Input: part model. Units: mm. Frame: model coordinates. A direction names the side the tool comes from. Coordinates: 2 decimals unless noted, no trailing zeros. Write each loop counter-clockwise with the first axis right and the second up, starting at its lowest first coordinate (ties: lowest second). Pieces come first, ordered by that corner, then holes. Notation, with made-up numbers: M 54,54.25 L 90,54.25 A25 ccw 90,81.25 Z; hole C 12.5,-5.75 d10. An arc over 180 degrees is marked long. Write each question's results on one line, items separated by ' | '. Start each with the question number.
1. First-contact query: pin 1 (4 mm diameter, centred on x = 10, y = -19, fed in from +Z); pin 2 (2.5 mm diameter, centred on x = 5.74, z = -24.03, fed in from -Y); pin 3 (8 mm diameter, centred on x = 16.5, y = -17.5, fed in from -Z); pin 4 (8 mm diameter, centred on y = -20.5, z = -42.5, fed in from +X). Flat tips, straight axial feed; report the tip coordinate or a pass-through.
2. Set-up query: faces 4 (the flat face through (-19.264, -17, -36)), 5 (the flat face through (0, -12, -35.632)), 6 (the flat face through (0, -14, -33.632)). Return all of +Z, -Z, +X, -X, +Y, -Y with unobstructed straight access to the full face (end or side cutting, diameter ignored); none if empty.
3. Pull-direction query (Z, two-part tool) for faces 1 (the flat face through (1, -26, -46)), 2 (the cylindrical face through (6.412, 0.986, -21.886)), 3 (the flat face through (-18.25, -20.93, -40.56)); classes: +Z half, -Z half, draft (parallel to the pull), parting line (faces both ways), or undercut.
4. Section query B-B, the plane y = -24.5. Output: boundary loops of the cut face in (x, z), and give its area (3 significant figures).
5. Section query A-A, the plane x = 7. Output: boundary loops of the cut face in (y, z).
6. Ray query, probe 1 along Z at (x, y) = (19, -14.25); probe 2 along Y at (x, z) = (-16, -45.5); probe 3 along Y at (x, z) = (3.5, -30). Return the intervals inside material, ascending.
7. Section query D-D, the plane z = -40. Output: boundary loops of the cut face in (x, y).
8. Section query C-C, the plane x = -1.5. Output: boundary loops of the cut face in (y, z).
```python
from build123d import *

# Parameters (mm, degrees)
SKETCH1_W           = 40
SKETCH1_H           = 100
SKETCH1_R           = 1.5
SKETCH1_R_2         = 2.25
BOSS_EXTRUDE1_DEPTH = 2
SKETCH2_W           = 40
SKETCH2_H           = 16
CUT_EXTRUDE1_DEPTH  = 10
SKETCH4_W           = 40
SKETCH4_H           = 2
BOSS_EXTRUDE2_DEPTH = 30
SKETCH5_W           = 40
SKETCH5_H           = 2
BOSS_EXTRUDE3_DEPTH = 20
SKETCH6_W           = 40
SKETCH6_H           = 2
BOSS_EXTRUDE4_DEPTH = 20
FILLET1_R           = 1
SKETCH7_R           = 1.5
CUT_EXTRUDE2_DEPTH  = 20
SKETCH8_R           = 1.5
CUT_EXTRUDE3_DEPTH  = 20
SKETCH9_R           = 2.25
CUT_EXTRUDE4_DEPTH  = 68.136662164
SKETCH10_W          = 1
SKETCH10_H          = 6.8
BOSS_EXTRUDE5_DEPTH = 2
BOSS_EXTRUDE6_START = -2
BOSS_EXTRUDE6_DEPTH = 2


with BuildPart() as part:
    # Sketch1 → Boss-Extrude1 (new body)
    with BuildSketch(Plane(origin=(0, 0, 0), x_dir=(1, 0, 0), z_dir=(0, 1, 0))):
        with Locations((0.735982487, -0.367991244)):
            Rectangle(SKETCH1_W, SKETCH1_H)
        with Locations(Location((-9.264017513, -40.367991244, 0), (0, 0, 270))):
            Circle(SKETCH1_R, mode=Mode.SUBTRACT)
        with Locations(Location((-4.264017513, -24.767991244, 0), (0, 0, 270))):
            Circle(SKETCH1_R_2, mode=Mode.SUBTRACT)
        with Locations(Location((10.735982487, -40.367991244, 0), (0, 0, 270))):
            Circle(SKETCH1_R, mode=Mode.SUBTRACT)
        with Locations(Location((5.735982487, -24.767991244, 0), (0, 0, 270))):
            Circle(SKETCH1_R_2, mode=Mode.SUBTRACT)
        with Locations(Location((-4.264017513, 24.032008756, 0), (0, 0, 270))):
            Circle(SKETCH1_R_2, mode=Mode.SUBTRACT)
        with Locations(Location((-9.264017513, 39.632008756, 0), (0, 0, 270))):
            Circle(SKETCH1_R, mode=Mode.SUBTRACT)
        Polygon((0.235982487, 26.632008756), (0.735982487, 26.632008756), (1.235982487, 26.632008756), (1.235982487, 19.832008756), (10.735982487, 19.832008756), (10.735982487, -20.567991244), (1.235982487, -20.567991244), (1.235982487, -27.367991244), (0.735982487, -27.367991244), (0.235982487, -27.367991244), (0.235982487, -20.567991244), (-9.264017513, -20.567991244), (-9.264017513, 19.832008756), (0.235982487, 19.832008756), align=None, mode=Mode.SUBTRACT)
        with Locations(Location((5.735982487, 24.032008756, 0), (0, 0, 270))):
            Circle(SKETCH1_R_2, mode=Mode.SUBTRACT)
        with Locations(Location((10.735982487, 39.632008756, 0), (0, 0, 270))):
            Circle(SKETCH1_R, mode=Mode.SUBTRACT)
    extrude(amount=BOSS_EXTRUDE1_DEPTH)

    # Sketch2 → Cut-Extrude1 (cut)
    with BuildSketch(Plane(origin=(0, 2, 0), x_dir=(1, 0, 0), z_dir=(0, 1, 0))):
        with Locations((0.735982487, 41.632008756)):
            Rectangle(SKETCH2_W, SKETCH2_H)
        with Locations((0.735982487, -42.367991244)):
            Rectangle(SKETCH2_W, SKETCH2_H)
    extrude(amount=-CUT_EXTRUDE1_DEPTH, mode=Mode.SUBTRACT)

    # Sketch4 → Boss-Extrude2 (add)
    with BuildSketch(Plane(origin=(0, 2, 0), x_dir=(1, 0, 0), z_dir=(0, 1, 0))):
        with Locations((0.735982487, -35.367991244)):
            Rectangle(SKETCH4_W, SKETCH4_H)
        with Locations((0.735982487, 34.632008756)):
            Rectangle(SKETCH4_W, SKETCH4_H)
    extrude(amount=-BOSS_EXTRUDE2_DEPTH)

    # Sketch5 → Boss-Extrude3 (add)
    with BuildSketch(Plane(origin=(0, 0, -35.632008756), x_dir=(-1, 0, 0), z_dir=(0, 0, -1))):
        with Locations((-0.735982487, -27)):
            Rectangle(SKETCH5_W, SKETCH5_H)
    extrude(amount=BOSS_EXTRUDE3_DEPTH)

    # Sketch6 → Boss-Extrude4 (add)
    with BuildSketch(Plane.XY.offset(36.367991244)):
        with Locations((0.735982487, -27)):
            Rectangle(SKETCH6_W, SKETCH6_H)
    extrude(amount=BOSS_EXTRUDE4_DEPTH)

    # Fillet1
    fillet1_edges = [part.edges().sort_by_distance(p)[0] for p in [
        (0.735982487, -28, 34.367991244),
        (0.735982487, 2, 36.367991244),
        (0.735982487, -28, -33.632008756),
        (0.735982487, 2, -35.632008756),
        (0.735982487, -26, -35.632008756),
        (0.735982487, -26, 36.367991244),
        (0.735982487, 0, 34.367991244),
        (0.735982487, 0, -33.632008756),
    ]]
    fillet(fillet1_edges, radius=FILLET1_R)

    # Sketch7 → Cut-Extrude2 (cut)
    with BuildSketch(Plane(origin=(0, -26, 0), x_dir=(1, 0, 0), z_dir=(0, 1, 0))):
        with Locations(Location((-9.264017513, 45.632008756, 0), (0, 0, 270))):
            Circle(SKETCH7_R)
        with Locations(Location((10.735982487, 45.632008756, 0), (0, 0, 270))):
            Circle(SKETCH7_R)
    extrude(amount=-CUT_EXTRUDE2_DEPTH, mode=Mode.SUBTRACT)

    # Sketch8 → Cut-Extrude3 (cut)
    with BuildSketch(Plane(origin=(0, -26, 0), x_dir=(1, 0, 0), z_dir=(0, 1, 0))):
        with Locations(Location((10.735982487, -46.367991244, 0), (0, 0, 270))):
            Circle(SKETCH8_R)
        with Locations(Location((-9.264017513, -46.367991244, 0), (0, 0, 270))):
            Circle(SKETCH8_R)
    extrude(amount=-CUT_EXTRUDE3_DEPTH, mode=Mode.SUBTRACT)

    # Sketch9 → Cut-Extrude4 (cut, through all)
    # profile 1 of 5: a face of its own
    with BuildSketch(Plane(origin=(0, 2, 0), x_dir=(1, 0, 0), z_dir=(0, 1, 0))):
        Polygon((36.675013235, 19.832008756), (20.735982487, 19.832008756), (20.735982487, -35.367991244), (10.735982487, -35.367991244), (10.735982487, -99.31179038), (10.735982487, -106.86631097), (36.675013235, -106.86631097), align=None)
    # profile 2 of 5: a face of its own
    with BuildSketch(Plane(origin=(0, 2, 0), x_dir=(1, 0, 0), z_dir=(0, 1, 0))):
        Polygon((10.735982487, -20.567991244), (10.735982487, 19.832008756), (1.235982487, 19.832008756), (0.235982487, 19.832008756), (-9.264017513, 19.832008756), (-9.264017513, -20.567991244), (0.235982487, -20.567991244), (0.235982487, -27.367991244), (1.235982487, -27.367991244), (1.235982487, -20.567991244), align=None)
    # profile 3 of 5: a face of its own
    with BuildSketch(Plane(origin=(0, 2, 0), x_dir=(1, 0, 0), z_dir=(0, 1, 0))):
        Polygon((10.735982487, -35.367991244), (10.735982487, -20.567991244), (1.235982487, -20.567991244), (1.235982487, -27.367991244), (0.235982487, -27.367991244), (0.235982487, -20.567991244), (-9.264017513, -20.567991244), (-9.264017513, 19.832008756), (-19.264017513, 19.832008756), (-19.264017513, -35.367991244), align=None)
        with Locations((-4.264017513, -24.767991244)):
            Circle(SKETCH9_R, mode=Mode.SUBTRACT)
        with Locations((5.735982487, -24.767991244)):
            Circle(SKETCH9_R, mode=Mode.SUBTRACT)
    # profile 4 of 5: a face of its own
    with BuildSketch(Plane(origin=(0, 2, 0), x_dir=(1, 0, 0), z_dir=(0, 1, 0))):
        Polygon((20.735982487, 19.832008756), (10.735982487, 19.832008756), (10.735982487, -20.567991244), (10.735982487, -35.367991244), (20.735982487, -35.367991244), align=None)
    # profile 5 of 5: a face of its own
    with BuildSketch(Plane(origin=(0, 2, 0), x_dir=(1, 0, 0), z_dir=(0, 1, 0))):
        Polygon((10.735982487, -99.31179038), (10.735982487, -35.367991244), (-19.264017513, -35.367991244), (-19.264017513, 19.832008756), (-32.318048619, 19.832008756), (-32.318048619, -99.31179038), align=None)
    extrude(amount=-CUT_EXTRUDE4_DEPTH, mode=Mode.SUBTRACT)

    # Sketch10 → Boss-Extrude5 (add)
    with BuildSketch(Plane(origin=(0, 2, 0), x_dir=(1, 0, 0), z_dir=(0, 1, 0))):
        with Locations((0.735982487, 23.232008756)):
            Rectangle(SKETCH10_W, SKETCH10_H)
    extrude(amount=-BOSS_EXTRUDE5_DEPTH)

    # Sketch11 → Boss-Extrude6 (add)
    with BuildSketch(Plane.ZY.offset(19.264017513).offset(BOSS_EXTRUDE6_START)):
        with BuildLine():
            Line((-35.632008756, -25), (-35.632008756, -16))
            Line((-35.632008756, -16), (-45.632008756, -26))
            Line((-45.632008756, -26), (-36.632008756, -26))
            ThreePointArc((-36.632008756, -26), (-37.339115537, -24.292893219), (-35.632008756, -25))
        make_face()
        with BuildLine():
            ThreePointArc((-36.632008756, -26), (-35.924901975, -25.707106781), (-35.632008756, -25))
            ThreePointArc((-35.632008756, -25), (-37.339115537, -24.292893219), (-36.632008756, -26))
        make_face()
    extrude(amount=BOSS_EXTRUDE6_DEPTH)


solid = part.part
```
Answer:
1) pin 1: z = -33.63 | pin 2: through | pin 3: z = -35.63 | pin 4: x = -17.26
2) face 4: +Z, -Z, -X, +Y, -Y | face 5: -Z, +X, +Y | face 6: +Z, +X, -X, -Y
3) face 1: draft | face 2: undercut | face 3: -Z half
4) outline: M -19.26,-44.13 L -17.26,-44.13 L -17.26,-35.63 L 20.74,-35.63 L 20.74,-33.63 L -19.26,-33.63 Z | area: 97.0 mm^2
5) outline: M -28,-55.63 L -26,-55.63 L -26,-36.63 A1 cw -25,-35.63 L 1,-35.63 A1 ccw 2,-34.63 L 2,-25.89 L 0,-25.89 L 0,-32.63 A1 cw -1,-33.63 L -27,-33.63 A1 ccw -28,-34.63 Z; M 0,-22.17 L 2,-22.17 L 2,-19.83 L 0,-19.83 Z
6) probe 1: -35.63 to -33.63 | probe 2: -28 to -26 | probe 3: 0 to 2
7) outline: M -19.26,-28 L 20.74,-28 L 20.74,-26 L -17.26,-26 L -17.26,-20.37 L -19.26,-20.37 Z
8) outline: M -28,-55.63 L -26,-55.63 L -26,-36.63 A1 cw -25,-35.63 L 1,-35.63 A1 ccw 2,-34.63 L 2,-19.83 L 0,-19.83 L 0,-32.63 A1 cw -1,-33.63 L -27,-33.63 A1 ccw -28,-34.63 Z
